Geometry: see drawing. Coordinates: mm, zero at the bounding-box minimum. A direction names the side the tool comes from. Round coordinates to 2 decimals unless told otherwise and drop trailing zeros. Write each loop counter-clockwise with the first axis right and the second up, starting at its lowest first coordinate (ties: lowest second). Pieces come first, ordered by that corner, then holes. Notation, with made-up numbers: M 41,-11 L 69,-11 A32 ccw 69,24 Z; hole C 6.5,21.5 d7. An arc over 180 degrees is marked long. Use a Markdown table: item, result.
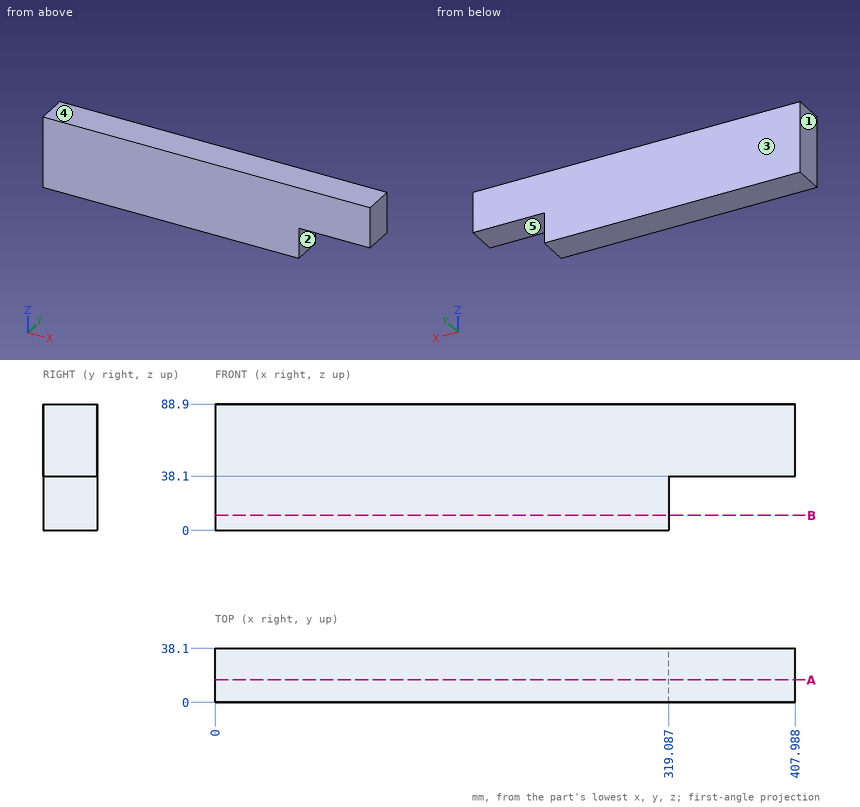
Q1. Line query: L1, parallel to X at y = 17.5, z = 9; L2, parallel to Z at x = 352, y = 12. Output: solid intervals per line, ascending.
Results are:
| item | result |
|---|---|
| L1 | 0 to 319.09 |
| L2 | 38.1 to 88.9 |
Q2. First-contact query: pin 1 Ø11.5 at (y, z) = (24.5, 12) entering from +X. Flat tip, straight axial feed; report the tip coordinate or a pass-through.
Results are:
| item | result |
|---|---|
| pin 1 | x = 319.09 |
Q3. Section B-B on z = 10.5. Return loops of the section in (x, y).
Results are:
| item | result |
|---|---|
| outline | M 0,0 L 319.09,0 L 319.09,38.1 L 0,38.1 Z |
Q4. Reachability of the marked faces 1 and 2 from +Z, -Z, +X, -X, +Y, -Y: full face, straight path, thin tool, end or side. Return the list, or none.
Results are:
| item | result |
|---|---|
| face 1 | +Z, -Z, -X, +Y, -Y |
| face 2 | -Z, +X, +Y, -Y |
Q5. Section A-A on y = 16. Return loops of the section in (x, z), plus the area to 3 significant figures.
Results are:
| item | result |
|---|---|
| outline | M 0,0 L 319.09,0 L 319.09,38.1 L 407.99,38.1 L 407.99,88.9 L 0,88.9 Z |
| area | 32,900 mm^2 |
Q6. Mould query, pull axis Z, two halves, no side actions, for the marked faces 3, 4 and 5. Classes: +Z half, -Z half, draft (parallel to the pull), parting line (faces both ways), or undercut.
Results are:
| item | result |
|---|---|
| face 3 | draft |
| face 4 | +Z half |
| face 5 | -Z half |
